Verification items for the finished model (mm, model axes). A direction names the side the tool comes from. Give positions to 0.01 mm unless a question says otherwise; leave off trailing zeros. Write each loop counter-clockwise with the first axis right and the second up, starting at its lowest first coordinate (ties: lowest second). Pieces come first, ordered by that corner, then holes. Notation, with made-up numbers: (37.5, 7.25) -> (64.5, 7.25) arc R24 ccw to (64.5, 31.25) -> close; hole circle Ø2 at (10, 27.25). An arc over 180 degrees is marked (long way). Use one line per item in the form item = value. Start each with the question number.
(1) Release check for a two-part mould opening along X. For faces 4 (the face through (1.81, 8.428, -1.107)), 5 (the face through (-2.5, 0, -4)), 6 (the face through (0.004, -3.955, -5.158)), 7 (the face through (6.636, -0.471, -4.309)) record: pulls with the +X half, pulls with the -X half, needs draft (parallel to the pull), parting line crosses it, or undercut.
(2) Set-up check for faces 1 (the face through (2.9, -2.8, 1.5)), 2 (the face through (4.27, 4.35, -0.05)), 3 (the face through (5.162, -5.857, 1.301)): record each of +Z, -Z, +X, -X, +Y, -Y from which the full face is reachable in a straight line by a thin tool's end or side.
(3) Section check D-D, the plane x = 1.75. Record the cut outline in (y, z) (3 decimals), plus the area to 3 significant figures.
(4) Section check A-A, the plane y = 0. State how many separate pieces and enclosed holes the cut face has, plus the area to 3 significant figures.
(5) Depth check by flat-ended pin: pin 1 Ø5.5 at (y, z) = (0, 0) entering from -X; pin 2 Ø1.5 at (x, z) = (5.5, 0) entering from -Y; pin 3 Ø2 at (y, z) = (5.5, -3.5) entering from +X; pin 4 Ø4 at (x, z) = (6.5, 5) entering from -Y. Enter the tip coordinate at first touch or a pass-through.
(6) Scan lines: L1, parallel to X at y = 3.95, z = 0; L2, parallel to X at y = 2, z = -6.25; L3, parallel to Z at x = 4.5, y = -1.5. Record each from-to range of solid material in increasing order.
from build123d import *

# Parameters (mm, degrees)
SKETCH2_R           = 6
BOSS_EXTRUDE1_DEPTH = 6
HOLE1_D             = 6.35
CHAMFER1_SIZE       = 0.6


# Read off the part's stored shape, not the designer's step: CSK for M2 Flat Head Machine Screw1, CSK for M2 Flat Head Machine Screw2
with BuildPart() as part:
    # Sketch1 → Revolve1 (revolve)
    with BuildSketch(Plane(origin=(0, 0, 0), x_dir=(-1, 0, 0), z_dir=(0, 0, -1)), mode=Mode.PRIVATE) as revolve1_sk:
        Polygon((-2.5, 8.5), (-2.5, 0), (2.5, 0), (2.5, 8.5), (1.1, 8.5), (0.271572875, 6.5), (-0.271572875, 6.5), (-1.1, 8.5), align=None)
    revolve(revolve1_sk.sketch.rotate(Axis((2.5, 0, 0), (-1, 0, 0)), 270), axis=Axis((2.5, 0, 0), (-1, 0, 0)))

    # Sketch2 → Boss-Extrude1 (add)
    with BuildSketch(Plane(origin=(2.5, 0, 0), x_dir=(0, 0, -1), z_dir=(1, 0, 0))):
        Circle(SKETCH2_R)
    extrude(amount=BOSS_EXTRUDE1_DEPTH)

    # Hole1 (through all)
    with Locations(Plane(origin=(8.5, 0, 0), x_dir=(0, 0, -1), z_dir=(1, 0, 0))):
        with Locations((0, 0)):
            Hole(HOLE1_D / 2)

    # CSK for M2 Flat Head Machine Screw1 outl → CSK for M2 Flat Head Machine Screw1 (revolve, cut)
    with BuildSketch(Plane(origin=(5.5, 0, 0), x_dir=(1, 0, 0), z_dir=(0, -1, 0))):
        Polygon((0, -6.000000161), (1.500000161, -6.000000161), (1.2295, -5.7295), (1.2295, -2.927170217), (0, -2.927170217), align=None)
    revolve(axis=Axis((5.5, 0, 0), (0, 0, 1)), mode=Mode.SUBTRACT)

    # CSK for M2 Flat Head Machine Screw2 outl → CSK for M2 Flat Head Machine Screw2 (revolve, cut)
    with BuildSketch(Plane(origin=(5.5, 0, 0), x_dir=(1, 0, 0), z_dir=(0, 0, 1))):
        Polygon((1.500065457, 6.000065457), (0, 6.000065457), (0, 2.927130581), (1.2295, 2.927130581), (1.2295, 5.7295), align=None)
    revolve(axis=Axis((5.5, 0, 0), (0, 1, 0)), mode=Mode.SUBTRACT)

    # Chamfer1
    chamfer1_edges = [part.edges().sort_by_distance(p)[0] for p in [
        (8.5, 0, 6),
    ]]
    chamfer(chamfer1_edges, length=CHAMFER1_SIZE)


solid = part.part
Completed:
q1.face_4 = needs draft
q1.face_5 = pulls with the -X half
q1.face_6 = undercut
q1.face_7 = undercut
q2.face_1 = +X, -X
q2.face_2 = +Y
q2.face_3 = +X
q3.outline = circle Ø17 at (0, 0); hole circle Ø6.35 at (0, 0)
q3.area = 195 mm²
q4.separate_pieces = 3
q4.enclosed_holes = 0
q4.area = 74.3 mm²
q5.pin_1 = through
q5.pin_2 = -6
q5.pin_3 = 8.38
q5.pin_4 = -5.2
q6.L1 = -2.5 to 4.27, 6.73 to 8.5
q6.L2 = -2.5 to -0.3, 0.3 to 2.5
q6.L3 = -5.81 to -2.8, 2.8 to 5.81
